Source: CAD feature listing. Evaluate the final solid. Frame: model axes, mm. A direction names the side the tool comes from. Give positions to 0.01 mm unless a question says otherwise; leave off trailing zeros. Order: outer loops, then holes, each group sorted by start corner. A loop starts at its lowest first (then second) coordinate and runs counter-clockwise, first axis right, second up.
from build123d import *

# Parameters (mm, degrees)
F0_W        = 10
F0_H        = 28.1
F0_R        = 1.4
F1_DEPTH    = 6
F0_H_2      = 6
F2_DEPTH    = 19.5
F0_H_3      = 6.2
F0_R_2      = 2.1
F3_DEPTH    = 12.5
F4_DEPTH    = 19.5
F5_DEPTH    = 12.5
F6_DEPTH    = 6.5
F7_T1_DEPTH = 55.8257569496
F8_S5_R     = 1.4
F8_T6_DEPTH = 5
F9_R        = 4
F10_SIZE    = 0.5


# Not quite as in the source:
# - a fillet or chamfer that OpenCascade refuses, or shapes differently, is made with other operations: its cross-section is extruded or revolved along the edge and cut away or added


with BuildPart() as f1:
    # F0 (on Top) → F1 (new body)
    with BuildSketch(Plane.XY):
        with Locations((-5, -11.2607904853)):
            Rectangle(F0_W, F0_H)
        with Locations((-4.5, -4.4107904853)):
            Circle(F0_R, mode=Mode.SUBTRACT)
    extrude(amount=F1_DEPTH)

    # F0 (on Top) → F2 (join)
    with BuildSketch(Plane.XY):
        with Locations((-5, -28.3107904853)):
            Rectangle(F0_W, F0_H_2)
    extrude(amount=F2_DEPTH)

    # F0 (on Top) → F3 (join)
    with BuildSketch(Plane.XY):
        with Locations((-5, -34.4107904853)):
            Rectangle(F0_W, F0_H_3)
        with Locations((-4.5, -34.4107904853)):
            Circle(F0_R_2, mode=Mode.SUBTRACT)
    extrude(amount=F3_DEPTH)

    # F0 (on Top) → F4 (join)
    with BuildSketch(Plane.XY):
        with Locations((-5, -40.5107904853)):
            Rectangle(F0_W, F0_H_2)
    extrude(amount=F4_DEPTH)

    # F0 (on Top) → F5 (join)
    with BuildSketch(Plane.XY):
        with Locations((-4.5, -34.4107904853)):
            Circle(F0_R_2)
        with Locations((-4.5, -34.4107904853)):
            Circle(F0_R, mode=Mode.SUBTRACT)
    extrude(amount=F5_DEPTH)

    # F0 (on Top) → F6 (cut)
    with BuildSketch(Plane.XY):
        with Locations((-4.5, -34.4107904853)):
            Circle(F0_R_2)
        with Locations((-4.5, -34.4107904853)):
            Circle(F0_R, mode=Mode.SUBTRACT)
    extrude(amount=F6_DEPTH, mode=Mode.SUBTRACT)

    # F7: fillet of radius 10 on 2 edges, made by hand

    # F7_s2 → F7_t1 (cut)
    with BuildSketch(Plane.YZ.offset(-32.9128784748)):
        with BuildLine():
            ThreePointArc((-31.3107904853, 19.5), (-26.9441902199, 15.8120741851), (-25.3107904853, 10.3348486101))
            Line((-25.3107904853, 10.3348486101), (-25.3107904853, 19.5))
            Line((-25.3107904853, 19.5), (-31.3107904853, 19.5))
        make_face()
        with BuildLine():
            ThreePointArc((-43.5107904853, 10.3348486101), (-41.8773907506, 15.8120741851), (-37.5107904853, 19.5))
            Line((-37.5107904853, 19.5), (-43.5107904853, 19.5))
            Line((-43.5107904853, 19.5), (-43.5107904853, 10.3348486101))
        make_face()
    extrude(amount=F7_T1_DEPTH, mode=Mode.SUBTRACT)

    # F8: chamfer of 2 on 1 edges, made by hand


with BuildPart() as f8_tool2:
    # F8_s3 → F8_t4 (revolve)
    with BuildSketch(Plane.XZ.offset(34.4107904853)):
        Polygon((-2.4, 4.5), (-4.4, 6.5), (-2.4, 6.5), align=None)
    revolve(axis=Axis((-4.5, -34.4107904853, 6.5), (0, 0, 1)))

    # F8_s5 → F8_t6 (cut, symmetric)
    with BuildSketch(Plane.XY.offset(5.5)):
        with Locations((-4.5, -34.4107904853)):
            Circle(F8_S5_R)
    extrude(amount=F8_T6_DEPTH, both=True, mode=Mode.SUBTRACT)


with BuildPart() as f1_1:
    add(f1.part)

    # F8_t1: union F8_tool2
    add(f8_tool2.part)

    # F9
    f9_edges = [f1_1.edges().sort_by_distance(p)[0] for p in [
        (-5, 2.78921, 6),
    ]]
    fillet(f9_edges, radius=F9_R)

    # F10
    f10_edges = [f1_1.edges().sort_by_distance(p)[0] for p in [
        (-5.9, -4.41079, 6),
    ]]
    chamfer(f10_edges, length=F10_SIZE)

    # F11: F1 across plane


with BuildPart() as f1_2:
    add(f1_1.part)
    add(f1_1.part.mirror(Plane.YZ))


solid = f1_2.part
1) Section query A-A on x = 4.5. Output: boundary loops of the cut face in (y, z), and give its area (3 significant figures).
Checks:
outline: (-43.51, 0) - (-36.51, 0) - (-36.51, 4.5) - (-35.81, 5.2) - (-35.81, 12.5) - (-37.51, 12.5) - (-37.51, 19.5) arc R10 ccw to (-43.51, 10.33) - close; (-33.01, 5.2) - (-32.31, 4.5) - (-32.31, 0) - (-5.81, 0) - (-5.81, 5.5) - (-6.31, 6) - (-25.31, 6) - (-25.31, 10.33) arc R10 ccw to (-31.31, 19.5) - (-31.31, 12.5) - (-33.01, 12.5) - close; (-3.01, 0) - (2.79, 0) - (2.79, 2) arc R4 ccw to (-1.21, 6) - (-2.51, 6) - (-3.01, 5.5) - close
area: 387 mm2
2) Reachability of faces 1 (the face through (10, -26, 5)), 2 (the face through (4.77, -32.33, 2.22)), 3 (the face through (0, -13, 6)) from +Z, -Z, +X, -X, +Y, -Y: full face, straight path, thin tool, end or side. Return the list, or none.
Checks:
face 1: +Z, -Z, +X, +Y, -Y
face 2: -Z
face 3: +Z, +X, -X, +Y
3) Section query C-C on z = 14.5. Output: boundary loops of the cut face in (x, y), and give its area (3 significant figures).
Checks:
outline: (-10, -42.6) - (10, -42.6) - (10, -37.51) - (-10, -37.51) - close; (-10, -31.31) - (10, -31.31) - (10, -26.22) - (-10, -26.22) - close
area: 204 mm2
4) First-contact query: pin 1 Ø2 at (x, z) = (4, 16) entering from +Y; pin 2 Ø2.5 at (x, y) = (4.5, -34.41) entering from -Z; pin 3 Ø5.5 at (x, z) = (-1.5, 15.5) entering from -Y; pin 4 Ø6 at (x, z) = (-4, 15) entering from -Y. Flat tips, straight axial feed; report the tip coordinate or a pass-through.
Checks:
pin 1: stops at y = -26.47
pin 2: passes through
pin 3: stops at y = -43.21
pin 4: stops at y = -43.37
5) Ray query, L1, parallel to Y at x = -4.5, z = 2.2; L2, parallel to Y at x = -4.5, z = 10.25; L3, parallel to Y at x = 4.5, z = 3.4. Return the intervals inside material, ascending.
Checks:
L1: y = -43.51 to -36.51, -32.31 to -5.81, -3.01 to 2.78
L2: y = -43.51 to -35.81, -33.01 to -25.31
L3: y = -43.51 to -36.51, -32.31 to -5.81, -3.01 to 2.54
6) Pull-direction query (Y, two-part tool) for faces 4 (the face through (0, -31.311, 16)), 5 (the face through (-10, -26, 5)), 6 (the face through (0, -34, 12.5)), 7 (the face through (0, -25.311, 8)); classes: +Y half, -Y half, draft (parallel to the pull), parting line (faces both ways), or undercut.
Checks:
face 4: undercut
face 5: draft
face 6: undercut
face 7: +Y half
7) Section query D-D on y = -14. Output: boundary loops of the cut face in (x, z), and give its area (3 significant figures).
Checks:
outline: (-10, 0) - (10, 0) - (10, 6) - (-10, 6) - close
area: 120 mm2
8) Section query B-B on x = 8.75. Output: boundary loops of the cut face in (y, z), and give its area (3 significant figures).
Checks:
outline: (-43.51, 0) - (2.79, 0) - (2.79, 2) arc R4 ccw to (-1.21, 6) - (-25.31, 6) - (-25.31, 10.33) arc R10 ccw to (-31.31, 19.5) - (-31.31, 12.5) - (-37.51, 12.5) - (-37.51, 19.5) arc R10 ccw to (-43.51, 10.33) - close
area: 446 mm2
